Geometry check sheet. Reference: the model listing, model coordinates, mm. A direction names the side the tool comes from. Give positions to 0.01 mm unless a question says otherwise; leave off trailing zeros. Write each loop counter-clockwise with the first axis right and the second up, starting at its lowest first coordinate (ties: lowest second). Pieces come first, ordered by that corner, then holes. Notation, with made-up numbers: (77, 67.25) - (99, 67.25) arc R21 cw to (99, 85.25) - close; hole circle Ø9 at (-35, -7.75). An arc over 180 degrees is marked (long way). Use a Markdown table: item, result.
```python
from build123d import *

# Parameters (mm, degrees)
SKETCH3_R           = 1
BOSS_EXTRUDE1_DEPTH = 1.5


with BuildPart() as part:
    # Sketch3 → Boss-Extrude1 (new, symmetric)
    with BuildSketch(Plane.XY):
        Polygon((-6, -7.5), (-6, 12.5), (-10, 12.5), (-10, -12.5), (10, -12.5), (10, 12.5), (6, 12.5), (6, -7.5), align=None)
        with Locations((-8, -2.5)):
            Circle(SKETCH3_R, mode=Mode.SUBTRACT)
        with Locations(Location((8, -2.5, 0), (0, 0, 180))):
            Circle(SKETCH3_R, mode=Mode.SUBTRACT)
    extrude(amount=BOSS_EXTRUDE1_DEPTH, both=True)


solid = part.part
```
1) Section check C-C on z = -0.75. Record the boundary of the cut face in (x, y), then the cut area to 3 significant figures.
Working result:
| item | result |
|---|---|
| outline | (-10, -12.5) - (10, -12.5) - (10, 12.5) - (6, 12.5) - (6, -7.5) - (-6, -7.5) - (-6, 12.5) - (-10, 12.5) - close; hole circle Ø2 at (-8, -2.5); hole circle Ø2 at (8, -2.5) |
| area | 254 mm² |
2) Mould release check, pull along Y, two halves, no side actions. Record for faces 3 (the flat face through (0, -12.5, 0)), 4 (the flat face through (10, 0, 0)), 5 (the cylindrical face through (-8.8, -3.1, 0)): pulls with the +Y half, pulls with the -Y half, needs draft (parallel to the pull), parting line crosses it, or undercut.
Working result:
| item | result |
|---|---|
| face 3 | pulls with the -Y half |
| face 4 | needs draft |
| face 5 | undercut |
3) Set-up check for faces 1 (the flat face through (0, -8, 1.5)), 2 (the flat face through (-6, 2, 0)): record each of +Z, -Z, +X, -X, +Y, -Y from which the full face is reachable in a straight line by a thin tool's end or side.
Working result:
| item | result |
|---|---|
| face 1 | +Z, +X, -X, +Y, -Y |
| face 2 | +Z, -Z, +Y |
4) Material ranges on L1, parallel to X at y = -6.25, z = -0.65; L2, parallel to Y at x = -8, z = 0.5; L3, parallel to Y at x = 0.5, z = -0.9, recorded low to high. Write a range as from..to.
Working result:
| item | result |
|---|---|
| L1 | x = -10..-6, 6..10 |
| L2 | y = -12.5..-3.5, -1.5..12.5 |
| L3 | y = -12.5..-7.5 |
5) Section check D-D on x = 8. Record the boundary of the cut face in (y, z).
Working result:
| item | result |
|---|---|
| outline | (-12.5, -1.5) - (-3.5, -1.5) - (-3.5, 1.5) - (-12.5, 1.5) - close; (-1.5, -1.5) - (12.5, -1.5) - (12.5, 1.5) - (-1.5, 1.5) - close |
6) Section check B-B on y = 5. Record the boundary of the cut face in (x, z).
Working result:
| item | result |
|---|---|
| outline | (-10, -1.5) - (-6, -1.5) - (-6, 1.5) - (-10, 1.5) - close; (6, -1.5) - (10, -1.5) - (10, 1.5) - (6, 1.5) - close |
7) Depth check by flat-ended pin: P1, Ø3, axis at x = 3.5, y = 4, coming from the -Z side. Enter the tip coordinate at first touch or a pass-through.
Working result:
| item | result |
|---|---|
| P1 | passes through |
8) Section check A-A on y = -2.5. Record the boundary of the cut face in (x, z), then the cut area to 3 significant figures.
Working result:
| item | result |
|---|---|
| outline | (-10, -1.5) - (-9, -1.5) - (-9, 1.5) - (-10, 1.5) - close; (-7, -1.5) - (-6, -1.5) - (-6, 1.5) - (-7, 1.5) - close; (6, -1.5) - (7, -1.5) - (7, 1.5) - (6, 1.5) - close; (9, -1.5) - (10, -1.5) - (10, 1.5) - (9, 1.5) - close |
| area | 12.0 mm² |
